Verification items for the finished model (mm, model axes). Face numbers are marked on the shaded views. A direction names the side the tool comes from. Coordinates: 2 decimals unless noted, no trailing zeros. Write each loop counter-clockwise with the first axis right and the second up, starting at its lowest first coordinate (ties: lowest second). Pieces come first, ordered by that corner, then holes. Notation, with made-up numbers: (18.25, 53) -> (47.25, 53) arc R18 cw to (47.25, 74) -> close; hole circle Ø7 at (11.25, 42). An arc over 180 degrees is marked (long way). Answer in a Markdown table with one row per item.
```python
from build123d import *

# Parameters (mm, degrees)
SKETCH1_W                                            = 52.54
SKETCH1_H                                            = 21
SKETCH1_R                                            = 2.5
BOSS_EXTRUDE1_DEPTH                                  = 45
SKETCH2_R                                            = 2
CUT_EXTRUDE1_DEPTH                                   = 57.179292448
SKETCH3_R                                            = 2
CUT_EXTRUDE2_DEPTH                                   = 5
CBORE_FOR_M2_5_HEX_SOCKET_HEAD_CAP_SCREW_D           = 2.9
CBORE_FOR_M2_5_HEX_SOCKET_HEAD_CAP_SCREW_CBORE_D     = 5.5
CBORE_FOR_M2_5_HEX_SOCKET_HEAD_CAP_SCREW_CBORE_DEPTH = 16
SKETCH6_R                                            = 3.1
CUT_EXTRUDE3_DEPTH                                   = 2
SKETCH7_W                                            = 33.04
SKETCH7_H                                            = 40.5
SKETCH7_R                                            = 14
BOSS_EXTRUDE2_DEPTH                                  = 1


with BuildPart() as part:
    # Sketch1 → Boss-Extrude1 (new body)
    with BuildSketch(Plane(origin=(0, 0, 0), x_dir=(1, 0, 0), z_dir=(0, 1, 0))):
        Rectangle(SKETCH1_W, SKETCH1_H)
        with Locations(Location((23.5, 0, 0), (0, 0, 90))):
            Circle(SKETCH1_R, mode=Mode.SUBTRACT)
        with Locations(Location((-23.5, 0, 0), (0, 0, 90))):
            Circle(SKETCH1_R, mode=Mode.SUBTRACT)
    extrude(amount=BOSS_EXTRUDE1_DEPTH)

    # Sketch2 → Cut-Extrude1 (cut, through all)
    with BuildSketch(Plane(origin=(0, 0, -10.5), x_dir=(-1, 0, 0), z_dir=(0, 0, -1))):
        with Locations((0, 23.75)):
            Circle(SKETCH2_R)
    extrude(amount=-CUT_EXTRUDE1_DEPTH, mode=Mode.SUBTRACT)

    # Sketch3 → Cut-Extrude2 (cut)
    with BuildSketch(Plane(origin=(0, 45, 0), x_dir=(1, 0, 0), z_dir=(0, 1, 0))):
        with Locations(Location((-14, 1.79, 0), (0, 0, 270))):
            Circle(SKETCH3_R)
        with Locations(Location((14, 1.79, 0), (0, 0, 270))):
            Circle(SKETCH3_R)
    extrude(amount=-CUT_EXTRUDE2_DEPTH, mode=Mode.SUBTRACT)

    # CBORE for M2.5 Hex Socket Head Cap Screw1 (through all)
    with Locations(Plane(origin=(-5.656854249, 18.093145751, -10.5), x_dir=(-1, 0, 0), z_dir=(0, 0, -1))):
        with Locations((0, 0), (-11.313708498, 0), (-11.313708498, 11.313708498), (0, 11.313708498)):
            CounterBoreHole(CBORE_FOR_M2_5_HEX_SOCKET_HEAD_CAP_SCREW_D / 2, CBORE_FOR_M2_5_HEX_SOCKET_HEAD_CAP_SCREW_CBORE_D / 2, CBORE_FOR_M2_5_HEX_SOCKET_HEAD_CAP_SCREW_CBORE_DEPTH)

    # Sketch6 → Cut-Extrude3 (cut)
    with BuildSketch(Plane(origin=(0, 45, 0), x_dir=(1, 0, 0), z_dir=(0, 1, 0))):
        with Locations(Location((0, -0.71, 0), (0, 0, 270))):
            Circle(SKETCH6_R)
    extrude(amount=-CUT_EXTRUDE3_DEPTH, mode=Mode.SUBTRACT)

    # Sketch7 → Boss-Extrude2 (add)
    with BuildSketch(Plane.XZ):
        with Locations((0, 30.75)):
            Rectangle(SKETCH7_W, SKETCH7_H)
        with Locations(Location((0, 30, 0), (0, 0, 270))):
            Circle(SKETCH7_R, mode=Mode.SUBTRACT)
    extrude(amount=-BOSS_EXTRUDE2_DEPTH)


solid = part.part
```
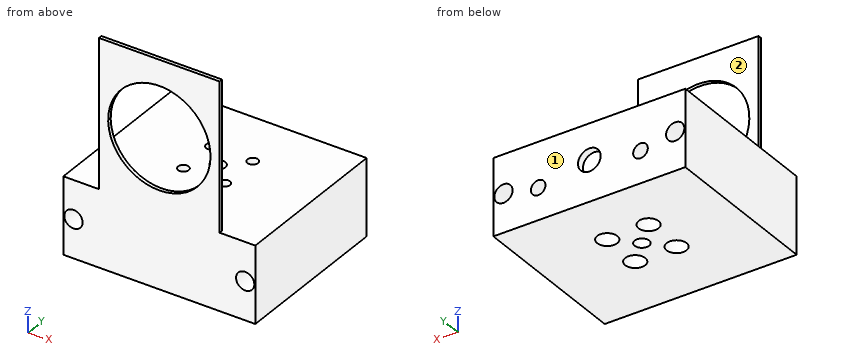
1. Sectioned sample at C-C, the plane y = 25. Record the cut outline in (x, z).
Findings below:
| item | result |
|---|---|
| outline | (-26.27, -10.5) -> (-1.56, -10.5) -> (-1.56, 10.5) -> (-26.27, 10.5) -> close; (1.56, -10.5) -> (26.27, -10.5) -> (26.27, 10.5) -> (1.56, 10.5) -> close; hole circle Ø5 at (-23.5, 0); hole circle Ø5 at (23.5, 0) |
2. Material ranges on probe 1 along X at (y, z) = (29.5, 6); probe 2 along Y at (x, z) = (0, 2.5); probe 3 along Y at (x, z) = (-5, -2), recorded low to high. Write a range as from..to.
Findings below:
| item | result |
|---|---|
| probe 1 | x = -26.27..-7.1, -4.21..4.21, 7.1..26.27 |
| probe 2 | y = 0..21.75, 25.75..43 |
| probe 3 | y = 0..15.42, 20.76..26.74, 32.08..45 |
3. Go/stop test with flat-tipped pins: pin 1 (10 mm diameter, centred on x = -5.5, y = 7, fed in from +Z); pin 2 (5 mm diameter, centred on x = -5.66, y = 18.09, fed in from -Z); pin 3 (10 mm diameter, centred on x = -17.5, z = 16.5, fed in from +Y). Record where each tip stops, or that it passes through.
Findings below:
| item | result |
|---|---|
| pin 1 | stops at z = 10.5 |
| pin 2 | stops at z = 5.5 |
| pin 3 | stops at y = 1 |
4. Sectioned sample at A-A, the plane z = 30. Record the cut outline in (x, y).
Findings below:
| item | result |
|---|---|
| outline | (-16.52, 0) -> (-14, 0) -> (-14, 1) -> (-16.52, 1) -> close; (14, 0) -> (16.52, 0) -> (16.52, 1) -> (14, 1) -> close |
5. Sectioned sample at D-D, the plane x = 23.5. Record the cut outline in (y, z), and give its area (3 significant figures).
Findings below:
| item | result |
|---|---|
| outline | (0, -10.5) -> (45, -10.5) -> (45, -2.5) -> (0, -2.5) -> close; (0, 2.5) -> (45, 2.5) -> (45, 10.5) -> (0, 10.5) -> close |
| area | 720 mm² |
6. Sectioned sample at B-B, the plane x = 0. Record the cut outline in (y, z), and give its area (3 significant figures).
Findings below:
| item | result |
|---|---|
| outline | (0, -10.5) -> (21.75, -10.5) -> (21.75, 10.5) -> (1, 10.5) -> (1, 16) -> (0, 16) -> close; (0, 44) -> (1, 44) -> (1, 51) -> (0, 51) -> close; (25.75, -10.5) -> (45, -10.5) -> (45, -2.39) -> (43, -2.39) -> (43, 3.81) -> (45, 3.81) -> (45, 10.5) -> (25.75, 10.5) -> close |
| area | 861 mm² |
7. Access from +Z, -Z, +X, -X, +Y, -Y to the whole of each face (thin tool, end or side, straight path). Record for the marked faces 1 and 2.
Findings below:
| item | result |
|---|---|
| face 1 | +Z, -Z, +X, -X, +Y |
| face 2 | +Z, +X, -X, +Y |
